Geometry: final body of the model. Coordinates: model frame, mm. Face numbers are marked on the shaded views. A direction names the side the tool comes from. Coordinates: 2 decimals unless noted, no trailing zeros. Order: outer loops, then holes, each group sorted by start corner. A loop starts at its lowest first (then second) coordinate and runs counter-clockwise, first axis right, second up. Notation, with made-up numbers: (7, -11.5) -> (15, -11.5) arc R21 cw to (15, 27.5) -> close; hole circle Ø5 at (85.5, -13). An arc over 180 degrees is marked (long way). Use one line per item in the form item = value.
```python
from build123d import *

# Parameters (mm, degrees)
F2_R = 1.22642
F3_R = 3.679261


with BuildPart() as f1:
    # F0 (on Front) → F1 (revolve)
    with BuildSketch(Plane.XZ):
        Polygon((0, 57.015903), (0, 0), (18.798783, 25.838224), (4.593469, 25.838224), (4.593469, 57.015903), align=None)
    revolve(axis=Axis((0, 0, 28.507952), (0, 0, 1)))

    # F2
    f2_edges = [f1.edges().sort_by_distance(p)[0] for p in [
        (-18.798783, 0, 25.838224),
        (-4.593469, 0, 25.838224),
    ]]
    fillet(f2_edges, radius=F2_R)

    # F3
    f3_edges = [f1.edges().sort_by_distance(p)[0] for p in [
        (-4.593469, 0, 57.015903),
    ]]
    fillet(f3_edges, radius=F3_R)


solid = f1.part
```
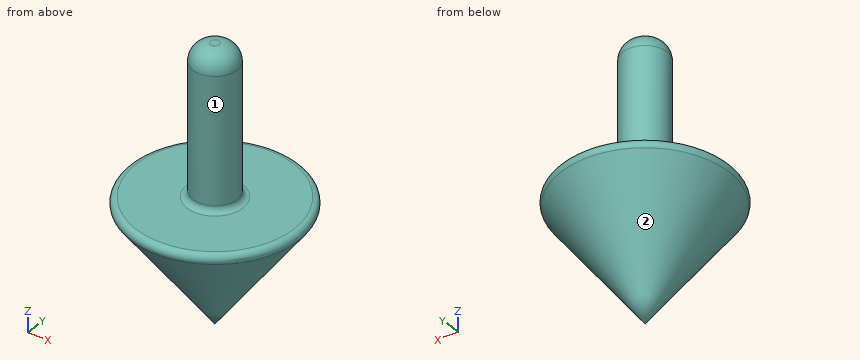
1) Access query for the marked faces 1 and 2. Directions: +Z, -Z, +X, -X, +Y, -Y. A direction counts if a zero-diameter tool reaches every point of the face in a straight line with its end or side. Return the directions, or none.
Results found:
face_1 = +Z
face_2 = -Z
2) Contact query for flat-ended pins moving along their axis: P1, Ø1.5, axis at y = -2, z = 29, coming from the -X side; P2, Ø6, axis at x = 0.5, z = 15, coming from the -Y side; P3, Ø12, axis at x = -13, y = -7, coming from the +Z side. Output: stop coordinate, or through.
Results found:
P1 = -4.42
P2 = -13.09
P3 = 25.84
3) Section A-A, the plane z = 29. Output: boundary loops of the cut face in (x, y), and give its area (3 significant figures).
Results found:
outline = circle Ø9.19 at (0, 0)
area = 66.3 mm2
4) Material intervals for probe 1 along Z at (x, y) = (-10.5, -14); probe 2 along Z at (x, y) = (-4.5, 11.5); probe 3 along X at (y, z) = (9.5, 15), sorted ascending. Write a range as from..to.
Results found:
probe_1 = 24.09..25.13
probe_2 = 16.97..25.84
probe_3 = -5.37..5.37
5) Section B-B, the plane z = 16. Output: boundary loops of the cut face in (x, y).
Results found:
outline = circle Ø23.28 at (0, 0)
